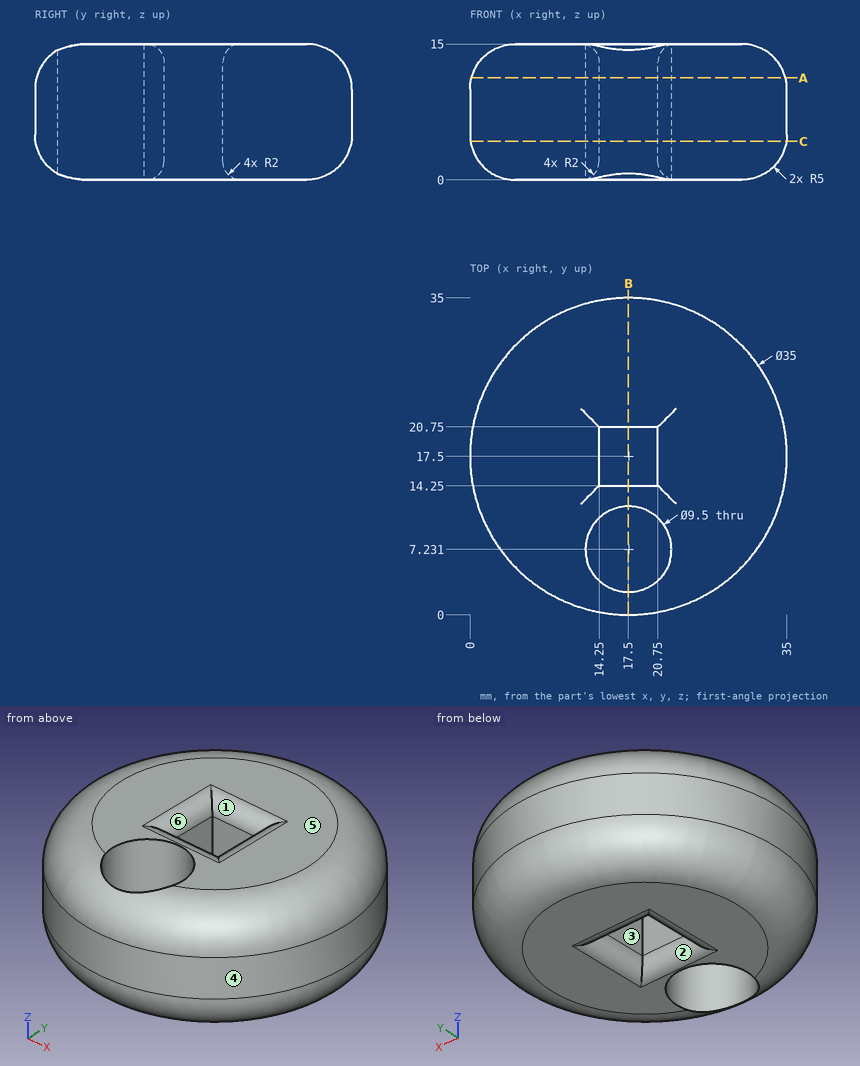
The figure shows three views and two pictorial views of one solid part (mm, origin at its lowest corner). Answer the questions. A direction names the side the tool comes from. Coordinates: 2 decimals unless noted, no trailing zeros. Loops run counter-clockwise (first coordinate to the right, second up) from the corner with the lowest first, then second, coordinate; pieces in that order, holes last. Notation, with made-up numbers: (12.5, 77) - (28.5, 77) arc R24 ccw to (28.5, 97) - close; hole circle Ø9 at (72, 56). An arc over 180 degrees is marked (long way). Answer in a Markdown table with one row per item.
Q1. Find section C-C on z = 4.25. Write down the section's boundary in (x, y), plus the area to 3 significant figures.
Here are the results:
| item | result |
|---|---|
| outline | circle Ø34.89 at (17.5, 17.5); hole circle Ø9.5 at (17.5, 7.23); hole (14.25, 14.25) - (20.75, 14.25) - (20.75, 20.75) - (14.25, 20.75) - close |
| area | 843 mm^2 |
Q2. Given P1, Ø4, axis at x = 13, z = 2.5, coming from the +Y side; P2, Ø2, axis at y = 10.5, z = 12.5, coming from the -X side; P3, Ø1, axis at y = 21.5, z = 12, coming from the +X side (1 decimal), each flat-ended and moving along its own axis, determine where each tip first touches the part or whether it passes through.
Here are the results:
| item | result |
|---|---|
| P1 | stops at y = 34.61 |
| P2 | stops at x = 1.53 |
| P3 | stops at x = 34.3 |
Q3. Find section A-A on z = 11.25. Write down the section's boundary in (x, y).
Here are the results:
| item | result |
|---|---|
| outline | circle Ø34.68 at (17.5, 17.5); hole circle Ø9.5 at (17.5, 7.23); hole (14.25, 14.25) - (20.75, 14.25) - (20.75, 20.75) - (14.25, 20.75) - close |
Q4. The mould has two halves that part along X. Classify the marked faces 4, 5 and 6: pulls with the +X half, pulls with the -X half, needs draft (parallel to the pull), parting line crosses it, or undercut.
Here are the results:
| item | result |
|---|---|
| face 4 | parting line crosses it |
| face 5 | needs draft |
| face 6 | undercut |
Q5. For the marked faces 1, 2 and 3, determine the directions among +Z, -Z, +X, -X, +Y, -Y from which every point of the face is accessible in a straight line to the end or side of a thin tool.
Here are the results:
| item | result |
|---|---|
| face 1 | +Z |
| face 2 | -Z |
| face 3 | +Z, -Z |
Q6. Find section B-B on x = 17.5. Count the separate pieces of the cut face and the enclosed holes in it, plus the area to 3 significant figures.
Here are the results:
| item | result |
|---|---|
| separate pieces | 3 |
| enclosed holes | 0 |
| area | 261 mm^2 |
Q7. Straight lines are drawn through the part: line 1 along Y through (x, z) = (17.5, 11); line 2 along X through (y, z) = (7, 13) (1 decimal); line 3 along X through (y, z) = (15.5, 10.5). For each, find the intervals that lie inside material, in ascending order. Write a range as [from, to].
Here are the results:
| item | result |
|---|---|
| line 1 | y = [0.1, 2.48], [11.98, 14.25], [20.75, 34.9] |
| line 2 | x = [4.8, 12.8], [22.2, 30.2] |
| line 3 | x = [0.14, 14.25], [20.75, 34.86] |
